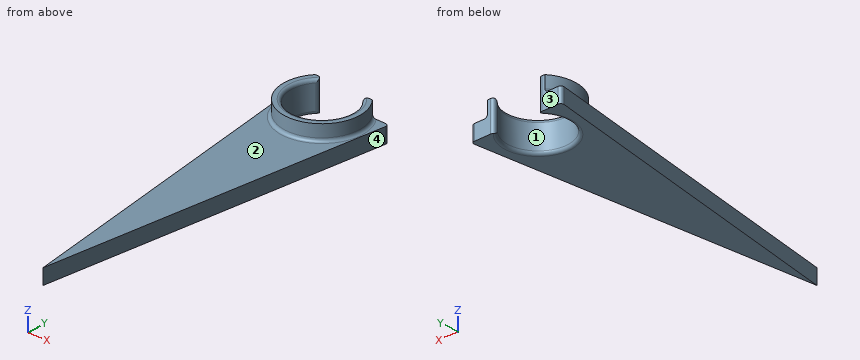
from build123d import *

# Parameters (mm, degrees)
F1_DEPTH = 5
F3_DEPTH = 5
F4_R     = 1


with BuildPart() as f1:
    # F0 (on Top) → F1 (new body)
    with BuildSketch(Plane.XY):
        with BuildLine():
            Line((-15, 0), (0, -110))
            Line((0, -110), (15, 0))
            Line((15, 0), (6, 0))
            ThreePointArc((6, 0), (8.94427191, -3.527864045), (10, -8))
            ThreePointArc((10, -8), (-4.472135955, -16.94427191), (-6, 0))
            Line((-6, 0), (-15, 0))
        make_face()
    extrude(amount=F1_DEPTH)

    # F2 (on face) → F3 (join)
    with BuildSketch(Plane.XY.offset(5)):
        with BuildLine():
            ThreePointArc((6, 0), (0, -18), (-6, 0))
            Line((-6, 0), (-9.4741754259, 0))
            ThreePointArc((-9.4741754259, 0), (0, -20.4), (9.4741754259, 0))
            Line((9.4741754259, 0), (6, 0))
        make_face()
    extrude(amount=F3_DEPTH)

    # F4
    f4_edges = [f1.edges().sort_by_distance(p)[0] for p in [
        (-6, 0, 5),
        (6, 0, 5),
        (0, -18, 10),
        (0, -18, 0),
        (0, -20.4, 5),
        (-15, 0, 2.5),
        (15, 0, 2.5),
    ]]
    fillet(f4_edges, radius=F4_R)


solid = f1.part
The listing builds one solid part. Answer for the finished solid, in the listing's coordinates (mm). Face numbers are marked on the shaded views. Round coordinates to 2 decimals unless told otherwise and drop trailing zeros. Order: outer loops, then holes, each group sorted by start corner. A loop starts at its lowest first (then second) coordinate and runs counter-clockwise, first axis right, second up. Notation, with made-up numbers: (-15.75, -35.5) -> (-1.75, -35.5) arc R27 ccw to (-1.75, -17.5) -> close; hole circle Ø2 at (-23, 8). An arc over 180 degrees is marked (long way). One line per item, written item: value.
Item 1: Find section C-C, the plane y = -63. Give the vertices of the cut face in (x, z), then the cut area to 3 significant figures.
Taken from the geometry:
outline: (-6.41, 0) -> (6.41, 0) -> (6.41, 5) -> (-6.41, 5) -> close
area: 64.1 mm2
Item 2: Find section B-B, the plane y = -97.5. Give the vertices of the cut face in (x, z), then the cut area to 3 significant figures.
Taken from the geometry:
outline: (-1.7, 0) -> (1.7, 0) -> (1.7, 5) -> (-1.7, 5) -> close
area: 17.0 mm2
Item 3: Given P1, Ø4, axis at y = -48, z = 4, coming from the +X side; P2, Ø3, axis at x = 1.5, y = -94, coming from the +Z side; P3, Ø1, axis at y = -81.5, z = 2, coming from the -X side, each flat-ended and moving along its own axis, determine where each tip first touches the part or whether it passes through.
Taken from the geometry:
P1: stops at x = 8.73
P2: stops at z = 5
P3: stops at x = -3.95
Item 4: For a pull along Y with two mould halves and no side action, classify the marked faces 1, 2, 3 and 4 as released by +Y, released by -Y, zero draft, split by the parting line, or undercut.
Taken from the geometry:
face 1: undercut
face 2: zero draft
face 3: released by +Y
face 4: released by -Y
Item 5: Find section A-A, the plane z = 3. Give the vertices of the cut face in (x, y), then the cut area to 3 significant figures.
Taken from the geometry:
outline: (-14.85, -1.14) -> (0, -110) -> (14.85, -1.14) arc R1 ccw to (13.85, 0) -> (8.49, 0) arc R1 ccw to (7.71, -1.64) arc R10 cw (long way) to (-7.71, -1.64) arc R1 ccw to (-8.49, 0) -> (-13.85, 0) arc R1 ccw to start
area: 1,350 mm2
Item 6: Straight lines are drawn through the part: L1, parallel to X at y = -8.5, z = 1; L2, parallel to Z at x = 2.75, y = -56; L3, parallel to X at y = -8, z = 7. For each, find the intervals that lie inside material, in ascending order.
Taken from the geometry:
L1: x = -13.84 to -9.99, 9.99 to 13.84
L2: z = 0 to 5
L3: x = -12.4 to -10, 10 to 12.4
